Autodesk Inventor part; units mm, degrees
ref_plane "YZ Plane" through (0, 0, 0) normal (1, 0, 0) x (0, 1, 0)
ref_plane "XZ Plane" through (0, 0, 0) normal (0, 1, 0) x (-1, 0, 0)
ref_plane "XY Plane" through (0, 0, 0) normal (0, 0, 1) x (1, 0, 0)
sketch "Sketch1" plane through (0, 0, 0) normal (0, 0, 1) x (1, 0, 0)
  line L0 (212.4649, 0) -> (106.2324, -184)
  line L1 (106.2324, -184) -> (-106.2324, -184)
  line L2 (-106.2324, -184) -> (-212.4649, 0)
  line L3 (-212.4649, 0) -> (-106.2324, 184)
  line L4 (-106.2324, 184) -> (106.2324, 184)
  line L5 (106.2324, 184) -> (212.4649, 0)
  point P0 (0, 0)
  point P1 (0, 0)
  dimension "d0" = 368
extrude "Extrusion1" add sketch "Sketch1" along normal blind 2
sketch "Sketch7" plane through (0, 0, 0) normal (0, 0, -1) x (-1, 0, 0)
  line L0 (-66.5995, 87.3368) -> (-66.5995, -40)
  line L1 (41.5995, 87.3368) -> (41.5995, -40)
  line L2 (-66.5995, -40) -> (41.5995, -40)
  arc A0 (41.5995, 87.3368) -> (-66.5995, 87.3368) centre (-12.5, 87.3368) ccw
  point P0 (0, 0)
extrude "Extrusion5" cut sketch "Sketch7" against normal blind 10
sketch "Sketch8" plane through (0, 0, 0) normal (0, 0, -1) x (-1, 0, 0)
  line L0 (-191.6803, 0) -> (-95.8401, 166)
  line L1 (-95.8401, 166) -> (96.1778, 166)
  line L2 (96.1778, 166) -> (191.5124, -0.2908)
  line L3 (191.5124, -0.2908) -> (95.8401, -166)
  line L4 (95.8401, -166) -> (-95.8401, -166)
  line L5 (-95.8401, -166) -> (-191.6803, 0)
  line L6 (-106.2324, -184) -> (-212.4649, 0)
  line L7 (-106.2324, -184) -> (-212.4649, 0)
  line L8 (106.2324, -184) -> (-106.2324, -184)
  line L9 (-106.2324, -184) -> (106.2324, -184)
  line L10 (212.4649, 0) -> (106.2324, -184)
  line L11 (106.2324, -184) -> (212.2788, -0.3224)
  line L12 (106.2324, 184) -> (212.4649, 0)
  line L13 (212.2788, -0.3224) -> (106.6066, 184)
  line L14 (-106.2324, 184) -> (106.2324, 184)
  line L15 (-106.2324, 184) -> (297.9127, 184)
  line L16 (-212.4649, 0) -> (-106.2324, 184)
  line L17 (-212.4649, 0) -> (-106.2324, 184)
  line L18 (-106.2324, 184) -> (106.2324, 184)
  point P0 (0, 0)
  dimension "d25" = 18
  dimension "d26" = 18
  dimension "d27" = 18
  dimension "d28" = 18
  dimension "d29" = 18
  dimension "d30" = 18
extrude "Extrusion6" cut sketch "Sketch8" against normal blind 1.25 contours L6 L16 L14 L12 L13 L10 L8 | L13 L12 L10
fillet "Fillet1" radius 5 6 edges at (-96.1778, 166, 0.625) (-191.5124, -0.2908, 0.625) (-95.8401, -166, 0.625) (95.8401, -166, 0.625) (191.6803, 0, 0.625) (95.8401, 166, 0.625)
sketch "Sketch10" plane through (0, 0, 0) normal (0, 0, -1) x (-1, 0, 0)
  circle A0 centre (13.7082, 139) radius 0.7835
  circle A1 centre (45.5995, 50.2789) radius 0.7835
  circle A2 centre (45.5995, -44) radius 0.7835
  circle A3 centre (-70.5995, -44) radius 0.7835
  circle A4 centre (-70.5995, 50.2789) radius 0.7835
  circle A5 centre (-38.7082, 139) radius 0.7835
  point P0 (0, 0)
extrude "Extrusion8" cut sketch "Sketch10" against normal blind 10
sketch "Sketch11" plane through (0, 0, 0) normal (0, 0, -1) x (-1, 0, 0)
  point P0 (0, 0)
sketch "Sketch12" plane through (0, 0, 2) normal (0, 0, 1) x (1, 0, 0)
  arc A0 (66.5995, 87.3368) -> (-41.5995, 87.3368) centre (12.5, 87.3368) ccw
  line L0 (-41.5995, -40) -> (-41.5995, 87.3368)
  line L1 (66.5995, 87.3368) -> (66.5995, -40)
  line L2 (66.5995, -40) -> (-41.5995, -40)
  arc A1 (67.0995, 87.3368) -> (-42.0995, 87.3368) centre (12.5, 87.3368) ccw
  line L3 (67.0995, 87.3368) -> (67.0995, -40.5)
  line L4 (67.0995, -40.5) -> (-42.0995, -40.5)
  line L5 (-42.0995, -40.5) -> (-42.0995, 87.3368)
  point P0 (0, 0)
  dimension "d35" = 0.5
extrude "Extrusion9" cut sketch "Sketch12" against normal blind 10 contours L1 L2 L0 A0 | L3 L4 L5 A1
sketch "Sketch13" plane through (0, 0, 2) normal (0, 0, 1) x (1, 0, 0)
  circle A0 centre (-13.7082, 139) radius 0.7835
  circle A1 centre (38.7082, 139) radius 0.7835
  circle A2 centre (70.5995, 50.2789) radius 0.7835
  circle A3 centre (-45.5995, 50.2789) radius 0.7835
  circle A4 centre (70.5995, -44) radius 0.7835
  circle A5 centre (-45.5995, -44) radius 0.7835
  point P0 (0, 0)
hole "Hole1" at (-45.5995, -44, 2) at (70.5995, -44, 2) at (70.5995, 50.2789, 2) at (-13.7082, 139, 2) at (38.7082, 139, 2) at (-45.5995, 50.2789, 2) direction (0, 0, -1) diameter 2.4 depth 3 tip angle 118 countersink diameter 4.4 countersink angle 90
equation "\"d26\" = d25"
equation "\"d27\" = d25"
equation "\"d28\" = d25"
equation "\"d29\" = d25"
equation "\"d30\" = d25"
properties part number "AEON.AluminiumFrame"
Geometry: final body of the model. Coordinates: model frame, mm. A direction names the side the tool comes from. Coordinates: 2 decimals unless noted, no trailing zeros. Order: outer loops, then holes, each group sorted by start corner. A loop starts at its lowest first (then second) coordinate and runs counter-clockwise, first axis right, second up. Notation, with made-up numbers: (5.25, -1) - (56.25, -1) arc R36 cw to (56.25, 38) - close; hole circle Ø4 at (-23, -4). An arc over 180 degrees is marked (long way). Write each question's results on one line, items separated by ' | '.
1) Section B-B, the plane x = -79. Return loops of the section in (y, z).
Results list:
outline: (-184, 1.25) - (-166, 1.25) - (-166, 0) - (166, 0) - (166, 1.25) - (184, 1.25) - (184, 2) - (-184, 2) - close
2) Line query: line 1 (X direction, y = -44, z = 0.4); line 2 (Y direction, x = 14.5, z = 0.8); line 3 (Z direction, x = 166.5, y = 49). Output: solid intervals per line, ascending. Write a range as from..to.
Results list:
line 1: -166.28..-46.8, -44.4..69.4, 71.8..166.28 | line 2: -166..-40.5, 141.9..166 | line 3: 1.25..2
3) Section D-D, the plane z = 0.4. Return loops of the section in (x, y), plus the area to 3 significant figures.
Results list:
outline: (-190.08, 2.2) arc R5 ccw to (-190.07, -2.78) - (-97.28, -163.5) arc R5 ccw to (-92.95, -166) - (92.95, -166) arc R5 ccw to (97.28, -163.5) - (190.24, -2.5) arc R5 ccw to (190.24, 2.5) - (97.28, 163.5) arc R5 ccw to (92.95, 166) - (-93.28, 166) arc R5 ccw to (-97.62, 163.49) - close; hole circle Ø2.4 at (-45.6, -44); hole circle Ø2.4 at (-45.6, 50.28); hole (-42.1, -40.5) - (67.1, -40.5) - (67.1, 87.34) arc R54.6 ccw to (-42.1, 87.34) - close; hole circle Ø2.4 at (-13.71, 139); hole circle Ø2.4 at (38.71, 139); hole circle Ø2.4 at (70.6, -44); hole circle Ø2.4 at (70.6, 50.28) | area: 76,800 mm^2
4) Pull-direction query (Y, two-part tool) for faces 4 (the cylindrical face through (13.701, 141.923, 1.014)), 5 (the flat face through (-144.328, -82.016, 0.616)), 6 (the flat face through (144.411, 81.873, 0.616)); classes: pulls with the +Y half, pulls with the -Y half, needs draft (parallel to the pull), parting line crosses it, or undercut.
Results list:
face 4: undercut | face 5: pulls with the -Y half | face 6: pulls with the +Y half
5) Section C-C, the plane y = -8.5. Return loops of the section in (x, z), plus the area to 3 significant figures.
Results list:
outline: (-207.56, 1.25) - (-186.77, 1.25) - (-186.77, 0) - (-42.1, 0) - (-42.1, 2) - (-207.56, 2) - close; (67.1, 0) - (186.77, 0) - (186.77, 1.25) - (207.56, 1.25) - (207.56, 2) - (67.1, 2) - close | area: 560 mm^2
6) Section A-A, the plane x = 12.5. Return loops of the section in (y, z), plus the area to 3 significant figures.
Results list:
outline: (-184, 1.25) - (-166, 1.25) - (-166, 0) - (-40.5, 0) - (-40.5, 2) - (-184, 2) - close; (141.94, 0) - (166, 0) - (166, 1.25) - (184, 1.25) - (184, 2) - (141.94, 2) - close | area: 326 mm^2
7) Pin query (flat end, axial travel): pin 1 (1 mm diameter, centred on y = 22.5, z = 1.5, fed in from +X); pin 2 (1.9 mm diameter, centred on x = -45.6, y = 50.28, fed in from -Z); pin 3 (3 mm diameter, centred on x = 38.71, y = 139, fed in from -Z); pin 4 (3 mm diameter, centred on x = -13.71, y = 139, fed in from +Z). Return the tip coordinate at first contact, or that it passes through.
Results list:
pin 1: x = 199.76 | pin 2: through | pin 3: z = 0 | pin 4: z = 1.3
8) Set-up query: faces 1 (the flat face through (-156, -67, 1.25)), 2 (the flat face through (143.11, -84.13, 0.62)), 3 (the flat face through (-143.203, 83.975, 0.616)). Return all of +Z, -Z, +X, -X, +Y, -Y with unobstructed straight access to the full face (end or side cutting, diameter ignored); none if empty.
Results list:
face 1: -Z | face 2: -Z, +X, -Y | face 3: -Z, -X, +Y
